Part model, mm, in its own coordinate system. Give positions to 0.01 mm unless a question says otherwise; leave off trailing zeros. Write each loop counter-clockwise with the first axis right and the second up, starting at its lowest first coordinate (ties: lowest second). Pieces come first, ordered by that corner, then holes. Notation, with made-up numbers: (-6.5, -32.75) - (39.5, -32.75) arc R30 ccw to (39.5, 6.25) - close; hole circle Ø2 at (21.25, 11). An arc over 180 degrees is marked (long way). Answer in a Markdown table with one row per item. Add a question column.
1. Band-saw the part on A-A on z = -11. Write the cut outline in (x, y), plus the area to 3 significant figures.
2. Band-saw the part on B-B on x = 63. Write the cut outline in (y, z), plus the area to 3 significant figures.
3. Probe line 1 along Z through (x, y) = (93, 2.8); line 2 along Z through (x, y) = (0, 2); line 3 along X through (y, z) = (5.1, -7). List the from-to ranges inside material, lowest first.
4. Band-saw the part on D-D on y = 0.9. State how many separate pieces and enclosed holes the cut face has, plus the area to 3 significant figures.
5. Band-saw the part on C-C on z = 11. Write the cut outline in (x, y).
Autodesk Inventor part; units mm, degrees
ref_plane "YZ Plane" through (0, 0, 0) normal (1, 0, 0) x (0, 1, 0)
ref_plane "XZ Plane" through (0, 0, 0) normal (0, 1, 0) x (-1, 0, 0)
ref_plane "XY Plane" through (0, 0, 0) normal (0, 0, 1) x (1, 0, 0)
sketch "Skizze1" plane through (0, 0, 0) normal (0, 1, 0) x (-1, 0, 0)
  line L0 (125, 75) -> (-125, 75)
  line L1 (-125, 75) -> (-125, -75)
  line L2 (-125, -75) -> (125, -75)
  line L3 (125, -75) -> (125, 75)
  point P0 (0, 0)
  point P1 (0, -75)
  point P2 (125, 0)
  dimension "d0" = 250
  dimension "d1" = 150
extrude "Extrusion1" add sketch "Skizze1" along normal blind 6
sketch "Skizze2" plane through (0, 0, 0) normal (0, -1, 0) x (1, 0, 0)
  circle A0 centre (0, -38) radius 12.5
  circle A1 centre (-93, -43) radius 9.5
  circle A2 centre (-93, -11) radius 9.5
  circle A3 centre (93, -43) radius 9.5
  circle A4 centre (93, -11) radius 9.5
  circle A5 centre (93, 43) radius 9.5
  circle A6 centre (-63, 43) radius 9.5
  circle A7 centre (63, 43) radius 9.5
  circle A8 centre (-93, 43) radius 9.5
  line L0 (125, 75) -> (125, -75)
  line L1 (-125, 75) -> (125, 75)
  line L2 (-125, -75) -> (-125, 75)
  line L3 (125, -75) -> (-125, -75)
  line L4 (-113, 63) -> (113, 63) construction
  line L5 (113, 63) -> (113, -63) construction
  line L6 (113, -63) -> (-113, -63) construction
  line L7 (-113, -63) -> (-113, 63) construction
  line L8 (-93, -11) -> (-93, -43) construction
  line L9 (93, -11) -> (93, -43) construction
  circle A9 centre (93, -43) radius 12.5 construction
  circle A10 centre (93, 43) radius 12.5 construction
  circle A11 centre (63, 43) radius 12.5 construction
  circle A12 centre (0, 43) radius 9.5
  circle A13 centre (0, 11) radius 9.5
  line L10 (0, 43) -> (0, 11) construction
  circle A14 centre (0, -38) radius 16 construction
  point P0 (0, 0)
  point P1 (93, -27)
  point P2 (-93, -27)
  point P3 (0, 10.7432)
  point P4 (0, -63)
  dimension "d4" = 25
  dimension "d5" = 19
  dimension "d6" = 19
  dimension "d7" = 19
  dimension "d8" = 19
  dimension "d9" = 19
  dimension "d10" = 19
  dimension "d11" = 19
  dimension "d12" = 19
  dimension "d13" = 12
  dimension "d14" = 12
  dimension "d15" = 12
  dimension "d16" = 12
  dimension "d19" = 32
  dimension "d20" = 20
  dimension "d21" = 20
  dimension "d22" = 20
  dimension "d23" = 25
  dimension "d25" = 20
  dimension "d26" = 25
  dimension "d27" = 25
  dimension "d28" = 30
  dimension "d30" = 30
  dimension "d33" = 32
  dimension "d34" = 25
extrude "Extrusion2" cut sketch "Skizze2" against normal through all contours A0 | A1 | A2 | A3 | A4 | A5 | A6 | A7 | A8 | A12 | A13
properties part number "Grundplatte_Konsole" material "Holz (Kirsche)"
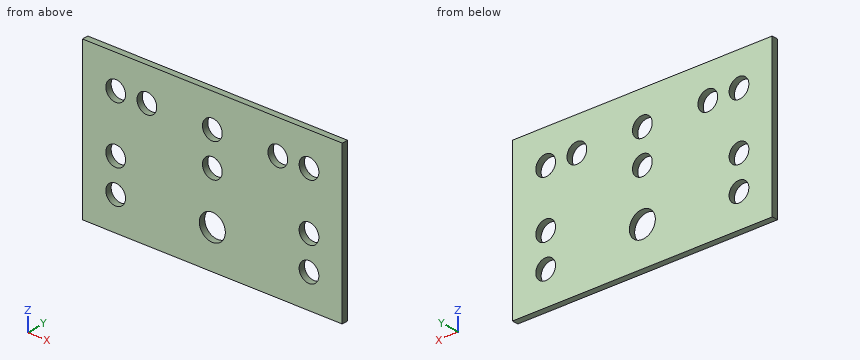
Values:
| question | item | result |
|---|---|---|
| 1 | outline | (-125, 0) - (-102.5, 0) - (-102.5, 6) - (-125, 6) - close; (-83.5, 0) - (83.5, 0) - (83.5, 6) - (-83.5, 6) - close; (102.5, 0) - (125, 0) - (125, 6) - (102.5, 6) - close |
| 1 | area | 1,270 mm² |
| 2 | outline | (0, -75) - (6, -75) - (6, 33.5) - (0, 33.5) - close; (0, 52.5) - (6, 52.5) - (6, 75) - (0, 75) - close |
| 2 | area | 786 mm² |
| 3 | line 1 | z = -75 to -52.5, -33.5 to -20.5, -1.5 to 33.5, 52.5 to 75 |
| 3 | line 2 | z = -75 to -50.5, -25.5 to 1.5, 20.5 to 33.5, 52.5 to 75 |
| 3 | line 3 | x = -125 to -101.62, -84.38 to 84.38, 101.62 to 125 |
| 4 | separate pieces | 1 |
| 4 | enclosed holes | 11 |
| 4 | area | 34,200 mm² |
| 5 | outline | (-125, 0) - (-9.5, 0) - (-9.5, 6) - (-125, 6) - close; (9.5, 0) - (125, 0) - (125, 6) - (9.5, 6) - close |
